from build123d import *

# Parameters (mm, degrees)
F0_W     = 40
F0_H     = 120
F1_DEPTH = 60
F2_W     = 34
F2_H     = 54
F3_DEPTH = 450
F5_DEPTH = 61


with BuildPart() as f1:
    # F0 (on Front) → F1 (new body)
    with BuildSketch(Plane.XZ):
        Rectangle(F0_W, F0_H)
    extrude(amount=F1_DEPTH)

    # F2 (on face) → F3 (cut)
    with BuildSketch(Plane(origin=(0, 0, -60), x_dir=(1, 0, 0), z_dir=(0, 0, -1))):
        with Locations((0, 30)):
            Rectangle(F2_W, F2_H)
    extrude(amount=-F3_DEPTH, mode=Mode.SUBTRACT)

    # F4 (on face) → F5 (cut)
    with BuildSketch(Plane.XZ.offset(60)):
        Polygon((20, 60), (-17, 60), (20, 23), align=None)
        Polygon((20, -60), (20, -23), (-17, -60), align=None)
    extrude(amount=-F5_DEPTH, mode=Mode.SUBTRACT)


solid = f1.part
For this review, take the finished solid that the model builds, in its own axes (mm). A direction names the side the tool comes from. Round coordinates to 2 decimals unless told otherwise and drop trailing zeros. Order: outer loops, then holes, each group sorted by start corner. A loop starts at its lowest first (then second) coordinate and runs counter-clockwise, first axis right, second up. Notation, with made-up numbers: (49, -35) -> (65, -35) arc R18 cw to (65, 0) -> close; hole circle Ø2 at (64.5, 43.5). An arc over 180 degrees is marked (long way). Write item = value, one per line. Start each with the question number.
1) To check wall thickness, follow line 1 (Y direction, x = -12, z = -1); line 2 (X direction, y = -13.5, z = -5); line 3 (X direction, y = -12.5, z = 31). State the ranges of each line that lie inside material, in increasing order. Write a range as from..to.
2) Insertion check: pin 1 (1.5 mm diameter, centred on x = 1.5, z = -42.5, fed in from +Y); pin 2 (4 mm diameter, centred on y = -38, z = 33.5, fed in from +X). Each pin has a flat end and moves straight along its axis. Give the tip position at first contact, or say it passes through.
3) Take a section at D-D on z = 15.5. State the section outline as (x, y) points.
4) Take a section at A-A on x = 1. State the section outline as (y, z) points, plus the area to 3 significant figures.
5) Tool access review of faces 1 (the face through (17, -30, 0)), 2 (the face through (18, -30, 25)): name each direction out of +Z, -Z, +X, -X, +Y, -Y from which nothing blocks a thin tool from reaching the whole face with its end or side.
6) Take a section at B-B on y = -18. State the section outline as (x, z) points, plus the area to 3 significant figures.
7) The part is to be moulded in two halves that separate along Y. For faces 3 (the face through (18, -30, -25)), 4 (the face through (-5, -60, 1)), 5 (the face through (-4, -57, -1)), say which applies: +Y half, -Y half, draft (parallel to the pull), parting line (faces both ways), or undercut.
8) Take a section at C-C on z = -30. State the section outline as (x, y) points.
Verdict:
q1.line_1 = -60..-57, -3..0
q1.line_2 = -20..-17, 17..20
q1.line_3 = -20..-17
q2.pin_1 = 0
q2.pin_2 = -17
q3.outline = (-20, -60) -> (20, -60) -> (20, 0) -> (-20, 0) -> close; hole (-17, -57) -> (17, -57) -> (17, -3) -> (-17, -3) -> close
q4.outline = (-60, -42) -> (-57, -42) -> (-57, 42) -> (-60, 42) -> close; (-3, -42) -> (0, -42) -> (0, 42) -> (-3, 42) -> close
q4.area = 504 mm2
q5.face_1 = +Z, -Z
q5.face_2 = +Z, +X, +Y, -Y
q6.outline = (-20, -60) -> (-17, -60) -> (-17, 60) -> (-20, 60) -> close; (17, -26) -> (20, -23) -> (20, 23) -> (17, 26) -> close
q6.area = 507 mm2
q7.face_3 = draft
q7.face_4 = -Y half
q7.face_5 = undercut
q8.outline = (-20, -60) -> (13, -60) -> (13, -57) -> (-17, -57) -> (-17, -3) -> (13, -3) -> (13, 0) -> (-20, 0) -> close
